from build123d import *

# Parameters (mm, degrees)
F0_W     = 15
F0_H     = 60
F0_R     = 3
F1_DEPTH = 8
F2_SIZE  = 0.3


with BuildPart() as f1:
    # F0 (on Top) → F1 (new body)
    with BuildSketch(Plane.XY):
        Rectangle(F0_W, F0_H)
        with Locations((0, -22.75)):
            Circle(F0_R, mode=Mode.SUBTRACT)
        with Locations((0, 22.75)):
            Circle(F0_R, mode=Mode.SUBTRACT)
    extrude(amount=F1_DEPTH)

    # F2
    f2_edges = [f1.edges().sort_by_distance(p)[0] for p in [
        (7.5, 0, 0),
        (0, 30, 0),
        (-7.5, 0, 0),
        (0, -30, 0),
        (-3, -22.75, 0),
        (-3, 22.75, 0),
    ]]
    chamfer(f2_edges, length=F2_SIZE)


solid = f1.part
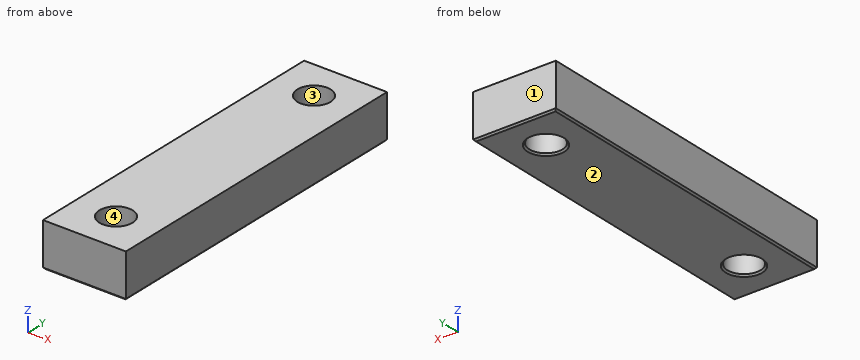
Build history of the part. All positions in model axes, mm. Face numbers are marked on the shaded views. Coordinates: 2 decimals unless noted, no trailing zeros. Order: outer loops, then holes, each group sorted by start corner. A loop starts at its lowest first (then second) coordinate and runs counter-clockwise, first axis right, second up. Notation, with made-up numbers: (-17, -26.75) - (16, -26.75) arc R19 ccw to (16, -9.75) - close; hole circle Ø1 at (14, 74). An arc over 180 degrees is marked (long way). Write item = value, one per line. Start each with the question number.
1) Wall check: line 1 along Y through (x, z) = (0, 4.5); line 2 along Y through (x, z) = (-2.25, 1.75); line 3 along X through (y, z) = (25, 7.5). Give the ranges that are in metal, low to high. Write a range as from..to.
2) Saw through at C-C on z = 6.75. Write the cut outline in (x, y), then the cut area to 3 significant figures.
3) Saw through at D-D on x = -2.5. Count the separate pieces of the cut face and the enclosed holes in it, then the cut area to 3 significant figures.
4) Saw through at B-B on x = 0. Write the cut outline in (y, z).
5) Saw through at A-A on y = 22.75. Write the cut outline in (x, z).
6) Two-plate mould, pull along Y, no slides. Class the marked faces 1, 2, 3 and 4: pulls with the +Y half, pulls with the -Y half, needs draft (parallel to the pull), parting line crosses it, or undercut.
From the geometry:
q1.line_1 = -30..-25.75, -19.75..19.75, 25.75..30
q1.line_2 = -30..-24.73, -20.77..20.77, 24.73..30
q1.line_3 = -7.5..-1.98, 1.98..7.5
q2.outline = (-7.5, -30) - (7.5, -30) - (7.5, 30) - (-7.5, 30) - close; hole circle Ø6 at (0, -22.75); hole circle Ø6 at (0, 22.75)
q2.area = 843 mm^2
q3.separate_pieces = 3
q3.enclosed_holes = 0
q3.area = 427 mm^2
q4.outline = (-30, 0.3) - (-29.7, 0) - (-26.05, 0) - (-25.75, 0.3) - (-25.75, 8) - (-30, 8) - close; (-19.75, 0.3) - (-19.45, 0) - (19.45, 0) - (19.75, 0.3) - (19.75, 8) - (-19.75, 8) - close; (25.75, 0.3) - (26.05, 0) - (29.7, 0) - (30, 0.3) - (30, 8) - (25.75, 8) - close
q5.outline = (-7.5, 0.3) - (-7.2, 0) - (-3.3, 0) - (-3, 0.3) - (-3, 8) - (-7.5, 8) - close; (3, 0.3) - (3.3, 0) - (7.2, 0) - (7.5, 0.3) - (7.5, 8) - (3, 8) - close
q6.face_1 = pulls with the +Y half
q6.face_2 = needs draft
q6.face_3 = undercut
q6.face_4 = undercut
